from build123d import *

# Parameters (mm, degrees)
SKETCH_R        = 6
PAD_DEPTH       = 30
PAD001_DEPTH    = 10
SKETCH002_R     = 1.75
HOLE_DEPTH      = 5
HOLE_TIPS_R     = 1.75
SKETCH003_R     = 3
POCKET_DEPTH    = 15
SKETCH004_R     = 2
POCKET001_DEPTH = 5


with BuildPart() as part:
    # Sketch → Pad (new body)
    with BuildSketch(Plane.XY):
        Circle(SKETCH_R)
    extrude(amount=PAD_DEPTH)

    # Sketch001 (on Face3 of Pad) → Pad001 (join)
    with BuildSketch(Plane.XY.offset(30)):
        Polygon((6.495191, -3.75), (6.495191, 3.75), (0, 7.5), (-6.495191, 3.75), (-6.495191, -3.75), (0, -7.5), align=None)
    extrude(amount=-PAD001_DEPTH)

    # Sketch002 (on Face11 of Pad001) → Hole (cut)
    with BuildSketch(Plane.XY.offset(30)):
        Circle(SKETCH002_R)
    extrude(amount=-HOLE_DEPTH, mode=Mode.SUBTRACT)

    # Hole tips → Hole tip 1 section 0
    with BuildSketch(Plane.XY.offset(25), mode=Mode.PRIVATE) as hole_tip_1_s0:
        Circle(HOLE_TIPS_R)
    loft([hole_tip_1_s0.sketch, Vertex(0, 0, 23.948494)], mode=Mode.SUBTRACT)

    # Sketch003 (on Face2 of Hole) → Pocket (cut)
    with BuildSketch(Plane(origin=(0, 0, 0), x_dir=(1, 0, 0), z_dir=(0, 0, -1))):
        Circle(SKETCH003_R)
    extrude(amount=-POCKET_DEPTH, mode=Mode.SUBTRACT)

    # Sketch004 (on DatumPlane) → Pocket001 (cut)
    with BuildSketch(Plane(origin=(0, 6, 10), x_dir=(1, 0, 0), z_dir=(0, -1, 0))):
        with Locations((0, -5)):
            Circle(SKETCH004_R)
    extrude(amount=POCKET001_DEPTH, mode=Mode.SUBTRACT)


solid = part.part
Part model, mm, in its own coordinate system. A direction names the side the tool comes from. Give positions to 0.01 mm unless a question says otherwise; leave off trailing zeros. Write each loop counter-clockwise with the first axis right and the second up, starting at its lowest first coordinate (ties: lowest second). Pieces come first, ordered by that corner, then holes.
1) Two-plate mould, pull along X, no slides. Class faces 5 (the face through (-2, -6, 20)), 6 (the face through (0.27, 0.08, 24.12)), 7 (the face through (3.202, -5.651, 25.07)): released by +X, released by -X, zero draft, split by the parting line, or undercut.
Resolved:
face 5: zero draft
face 6: undercut
face 7: released by +X
2) Cut at D-D on z = 5. Write the cut outline in (x, y), then the cut area to 3 significant figures.
Resolved:
outline: (-2, 2.24) - (-2, 5.66) arc R6 ccw (long way) to (2, 5.66) - (2, 2.24) arc R3 cw (long way) to start
area: 72.3 mm2
3) Pin check, flat tips, straight feed: pin 1 (3 mm diameter, centred on x = 0, y = 0, fed in from -Z); pin 2 (3 mm diameter, centred on x = -2.5, z = 21, fed in from +Y); pin 3 (5 mm diameter, centred on x = 2, z = 6, fed in from +Y). Stop position of each tip, or through.
Resolved:
pin 1: stops at z = 15
pin 2: stops at y = 6.92
pin 3: stops at y = 6
4) Cut at A-A on z = 14.5. Write the cut outline in (x, y), then the cut area to 3 significant figures.
Resolved:
outline: circle Ø12 at (0, 0); hole circle Ø6 at (0, 0)
area: 84.8 mm2
5) Probe L1, parallel to Y at x = 0, z = 7.75; L2, parallel to Z at x = 0, y = 3.5; L3, parallel to Z at x = 1.5, y = -2.5. List the from-to ranges inside material, lowest first.
Resolved:
L1: y = -6 to -3, 3 to 6
L2: z = 0 to 3, 7 to 30
L3: z = 15 to 30
6) Which spindle directions (+Z, -Z, +X, -X, +Y, -Y) get a long thin tool onto all of the face, cutting with end or side? Do faces 1 (the face through (1.847, 4.145, 4.234)), 2 (the face through (3.29, 5.6, 25.07)), 3 (the face through (1.617, -0.67, 27.535)), 4 (the face through (0, -3, 7)). Say none if no direction does.
Resolved:
face 1: +Y
face 2: +Z, -Z, +X, +Y
face 3: +Z
face 4: -Z
7) Cut at C-C on y = -4.5. Write the cut outline in (x, z).
Resolved:
outline: (-5.2, 20) - (-3.97, 20) - (-3.97, 0) - (3.97, 0) - (3.97, 20) - (5.2, 20) - (5.2, 30) - (-5.2, 30) - close
8) Cut at B-B on x = 5.25. Write the cut outline in (y, z), then the cut area to 3 significant figures.
Resolved:
outline: (-4.47, 20) - (-2.9, 20) - (-2.9, 0) - (2.9, 0) - (2.9, 20) - (4.47, 20) - (4.47, 30) - (-4.47, 30) - close
area: 206 mm2
